from build123d import *

# Parameters (mm, degrees)
SKETCH_1_W          = 60
SKETCH_1_H          = 15
EXTRUDE_1_DEPTH     = 450
SKETCH_2_R          = 3
CUT_EXTRUDE_1_DEPTH = 452.061248613
CUT_EXTRUDE_2_DEPTH = 452.061248613
SKETCH_4_W          = 36.3
SKETCH_4_H          = 7
CUT_EXTRUDE_3_DEPTH = 452.061248613
FILLET_1_R          = 2
CUT_EXTRUDE_4_DEPTH = 452.248268695


with BuildPart() as part:
    # 스케치1 → 보스-돌출1 (new body)
    with BuildSketch(Plane.XY):
        Rectangle(SKETCH_1_W, SKETCH_1_H)
    extrude(amount=EXTRUDE_1_DEPTH)

    # 스케치2 → 컷-돌출1 (cut, through all)
    with BuildSketch(Plane(origin=(0, 0, 0), x_dir=(-1, 0, 0), z_dir=(0, 0, -1))):
        with Locations((-25, -2.5)):
            Circle(SKETCH_2_R)
        with Locations((25, -2.5)):
            Circle(SKETCH_2_R)
    extrude(amount=-CUT_EXTRUDE_1_DEPTH, mode=Mode.SUBTRACT)

    # 스케치3 → 컷-돌출2 (cut, through all)
    with BuildSketch(Plane(origin=(0, 0, 0), x_dir=(-1, 0, 0), z_dir=(0, 0, -1))):
        with BuildLine():
            Line((-22.171572875, -6), (22.171572875, -6))
            ThreePointArc((22.171572875, -6), (20.939339828, -4.439339828), (20.5, -2.5))
            Line((20.5, -2.5), (25, -2.5))
            Line((25, -2.5), (25, 0.5))
            Line((25, 0.5), (-25, 0.5))
            Line((-25, 0.5), (-25, -2.5))
            Line((-25, -2.5), (-20.5, -2.5))
            ThreePointArc((-20.5, -2.5), (-20.939339828, -4.439339828), (-22.171572875, -6))
        make_face()
    extrude(amount=-CUT_EXTRUDE_2_DEPTH, mode=Mode.SUBTRACT)

    # 스케치4 → 컷-돌출3 (cut, through all)
    with BuildSketch(Plane(origin=(0, 0, 0), x_dir=(-1, 0, 0), z_dir=(0, 0, -1))):
        with Locations((0.006888359, 4)):
            Rectangle(SKETCH_4_W, SKETCH_4_H)
    extrude(amount=-CUT_EXTRUDE_3_DEPTH, mode=Mode.SUBTRACT)

    # 필렛1
    fillet_1_edges = [part.edges().sort_by_distance(p)[0] for p in [
        (-18.156888359, 0.5, 225),
        (18.143111641, 0.5, 225),
    ]]
    fillet(fillet_1_edges, radius=FILLET_1_R)

    # 스케치5 → 컷-돌출4 (cut, through all)
    with BuildSketch(Plane.XZ.offset(7.5)):
        Polygon((30, 450), (0, 450), (30, 420), align=None)
        Polygon((0, 450), (-30, 450), (-30, 420), align=None)
        Polygon((0, 0), (-30, 30), (-30, 0), align=None)
        Polygon((30, 30), (0, 0), (30, 0), align=None)
    extrude(amount=-CUT_EXTRUDE_4_DEPTH, mode=Mode.SUBTRACT)


solid = part.part
The model under review builds one solid part; all positions refer to its coordinate system, in mm. Round coordinates to 2 decimals unless told otherwise and drop trailing zeros. Order: outer loops, then holes, each group sorted by start corner. A loop starts at its lowest first (then second) coordinate and runs counter-clockwise, first axis right, second up. Notation, with made-up numbers: (66.5, -18) -> (74.5, -18) arc R13 ccw to (74.5, 5) -> close; hole circle Ø6 at (58, -9.5). An arc over 180 degrees is marked (long way). Write item = value, one per line. Start each with the question number.
Item 1: For line 1 along Y through (x, z) = (-25, 298); line 2 along X through (y, z) = (2.75, 293); line 3 along X through (y, z) = (-4.25, 206.5), list the stretches that pass through material, from the lowest coordinate up.
Item 2: Consider section A-A on z = 303.5. Write out the cut boundary in (x, y).
Item 3: Consider section B-B on x = -7. Write out the cut boundary in (y, z), plus the area to 3 significant figures.
Item 4: Clearance check with flat-ended pins moving along their axes: pin 1 Ø2 at (x, z) = (-16.5, 73.5) entering from +Y; pin 2 Ø7 at (x, y) = (-25, -2.5) entering from -Z; pin 3 Ø8 at (x, y) = (25, -2.5) entering from -Z. State where each tip first meets the part, or that it passes through.
Item 5: Mouldability with a two-part tool opening along X and no side actions: class faces 1 (the face through (22, 2, 22)), 2 (the face through (0, -7.5, 222)), 3 (the face through (0, -6, 222)) as released by +X, released by -X, zero draft, split by the parting line, or undercut.
Conclusion:
q1.line_1 = -7.5 to -5.5, 0.5 to 7.5
q1.line_2 = -30 to -18.16, 18.14 to 30
q1.line_3 = -30 to -27.44, -22.56 to -20.85, 20.85 to 22.56, 27.44 to 30
q2.outline = (-30, -7.5) -> (30, -7.5) -> (30, 7.5) -> (18.14, 7.5) -> (18.14, 2.5) arc R2 ccw to (20.14, 0.5) -> (25, 0.5) arc R3 cw (long way) to (22, -2.5) -> (20.5, -2.5) arc R4.5 ccw to (22.17, -6) -> (-22.17, -6) arc R4.5 ccw to (-20.5, -2.5) -> (-22, -2.5) arc R3 cw (long way) to (-25, 0.5) -> (-20.16, 0.5) arc R2 ccw to (-18.16, 2.5) -> (-18.16, 7.5) -> (-30, 7.5) -> close
q3.outline = (-7.5, 7) -> (-6, 7) -> (-6, 443) -> (-7.5, 443) -> close
q3.area = 654 mm2
q4.pin_1 = -6
q4.pin_2 = 21.5
q4.pin_3 = 21
q5.face_1 = released by +X
q5.face_2 = zero draft
q5.face_3 = undercut
